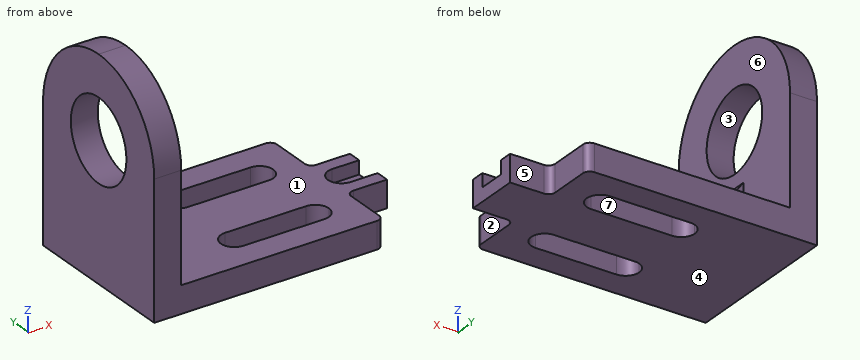
```python
from build123d import *

# Parameters (mm, degrees)
F1_DEPTH = 25.4
F2_DEPTH = 12.7
F3_R     = 38.1
F4_DEPTH = 25.4
F6_START = -63.5
F6_DEPTH = 25.4


with BuildPart() as f1:
    # F0 (on Top) → F1 (new body)
    with BuildSketch(Plane.XY):
        with BuildLine():
            Line((88.9, -38.1), (0, -38.1))
            Line((0, -38.1), (0, -114.3))
            Line((0, -114.3), (88.9, -114.3))
            ThreePointArc((88.9, -114.3), (92.6197438789, -105.3197438789), (101.6, -101.6))
            Line((101.6, -101.6), (177.8, -101.6))
            ThreePointArc((177.8, -101.6), (186.7802561211, -105.3197438789), (190.5, -114.3))
            Line((190.5, -114.3), (215.9, -114.3))
            Line((215.9, -114.3), (215.9, -107.95))
            ThreePointArc((215.9, -107.95), (217.7598719395, -103.4598719395), (222.25, -101.6))
            Line((222.25, -101.6), (254, -101.6))
            Line((254, -101.6), (254, -88.9))
            Line((254, -88.9), (228.6, -88.9))
            ThreePointArc((228.6, -88.9), (219.6197438789, -85.1802561211), (215.9, -76.2))
            ThreePointArc((215.9, -76.2), (219.6197438789, -67.2197438789), (228.6, -63.5))
            Line((228.6, -63.5), (254, -63.5))
            Line((254, -63.5), (254, -50.8))
            Line((254, -50.8), (222.25, -50.8))
            ThreePointArc((222.25, -50.8), (217.7598719395, -48.9401280605), (215.9, -44.45))
            Line((215.9, -44.45), (215.9, -38.1))
            Line((215.9, -38.1), (190.5, -38.1))
            ThreePointArc((190.5, -38.1), (186.7802561211, -47.0802561211), (177.8, -50.8))
            Line((177.8, -50.8), (101.6, -50.8))
            ThreePointArc((101.6, -50.8), (92.6197438789, -47.0802561211), (88.9, -38.1))
        make_face()
        with BuildLine():
            Line((209.55, 0), (0, 0))
            Line((0, 0), (0, -38.1))
            Line((0, -38.1), (88.9, -38.1))
            ThreePointArc((88.9, -38.1), (92.6197438789, -29.1197438789), (101.6, -25.4))
            Line((101.6, -25.4), (177.8, -25.4))
            ThreePointArc((177.8, -25.4), (186.7802561211, -29.1197438789), (190.5, -38.1))
            Line((190.5, -38.1), (215.9, -38.1))
            Line((215.9, -38.1), (215.9, -6.35))
            ThreePointArc((215.9, -6.35), (214.0401280605, -1.8598719395), (209.55, 0))
        make_face()
        with BuildLine():
            Line((88.9, -114.3), (0, -114.3))
            Line((0, -114.3), (0, -152.4))
            Line((0, -152.4), (209.55, -152.4))
            ThreePointArc((209.55, -152.4), (214.0401280605, -150.5401280605), (215.9, -146.05))
            Line((215.9, -146.05), (215.9, -114.3))
            Line((215.9, -114.3), (190.5, -114.3))
            ThreePointArc((190.5, -114.3), (186.7802561211, -123.2802561211), (177.8, -127))
            Line((177.8, -127), (101.6, -127))
            ThreePointArc((101.6, -127), (92.6197438789, -123.2802561211), (88.9, -114.3))
        make_face()
    extrude(amount=F1_DEPTH)

    # F0 (on Top) → F2 (join)
    with BuildSketch(Plane.XY):
        with BuildLine():
            Line((254, -88.9), (254, -63.5))
            Line((254, -63.5), (228.6, -63.5))
            ThreePointArc((228.6, -63.5), (219.6197438789, -67.2197438789), (215.9, -76.2))
            ThreePointArc((215.9, -76.2), (219.6197438789, -85.1802561211), (228.6, -88.9))
            Line((228.6, -88.9), (254, -88.9))
        make_face()
    extrude(amount=F2_DEPTH)

    # F3 (on face) → F4 (join)
    with BuildSketch(Plane(origin=(0, 0, 0), x_dir=(0, -1, 0), z_dir=(-1, 0, 0))):
        with BuildLine():
            Line((0, 127), (0, 25.4))
            Line((0, 25.4), (152.4, 25.4))
            Line((152.4, 25.4), (152.4, 127))
            ThreePointArc((152.4, 127), (130.0815367264, 180.8815367264), (76.2, 203.2))
            ThreePointArc((76.2, 203.2), (22.3184632736, 180.8815367264), (0, 127))
        make_face()
        with Locations((76.2, 127)):
            Circle(F3_R, mode=Mode.SUBTRACT)
    extrude(amount=-F4_DEPTH)

    # F5 (on face) → F6 (join)
    with BuildSketch(Plane.XZ.offset(152.4).offset(F6_START)):
        Polygon((25.4, 76.2), (25.4, 25.4), (63.5, 25.4), align=None)
    extrude(amount=-F6_DEPTH)


solid = f1.part
```
Can you work these out from the model? Positions are in its coordinate system, mm. Face numbers are marked on the shaded views. A direction names the side the tool comes from. Round coordinates to 2 decimals unless told otherwise and drop trailing zeros. Loops run counter-clockwise (first coordinate to the right, second up) from the corner with the lowest first, then second, coordinate; pieces in that order, holes last. Notation, with made-up numbers: M 42,47.5 L 49,47.5 A18 ccw 49,76.5 Z; hole C -32.75,42.25 d5. An arc over 180 degrees is marked long. Answer as a JSON object with one key per item and string values. Group by question number.
Q1. Will these pins go through, and if not, where does the flat tip stop? pin 1 (12.5 mm diameter, centred on y = -28.5, z = 9, fed in from +X); pin 2 (10 mm diameter, centred on x = 245, z = 18, fed in from +Y); pin 3 (20.5 mm diameter, centred on x = 246, z = 15, fed in from -Y).
Q2. Imagine slicing it at B-B, the plane z = 41. Please give me the cut outline in (x, y), then the cut area to 3 significant figures.
Q3. Imagine slicing it at D-D, the plane z = 117. Please give me the cut outline in (x, y), then the cut area to 3 significant figures.
Q4. We'd pull the mould along Z, two halves only. Please class the marked faces 1, 2, 3 and 4: +Z half, -Z half, draft (parallel to the pull), parting line (faces both ways), or undercut.
Q5. Please list where these lines run through material, in increasing order: L1, parallel to Z at x = 8, y = -76; L2, parallel to X at y = -118, z = 173.5; L3, parallel to Z at x = 223.5, y = -67.5.
Q6. Imagine slicing it at A-A, the plane z = 19. Please give me the cut outline in (x, y).
Q7. Imagine slicing it at C-C, the plane x = 187.5. Please give me the cut outline in (y, z).
Q8. On a 3-axis mill with a long thin cutter (end or side, diameter ignored), from which of +Z, -Z, +X, -X, +Y, -Y can I reach the whole of each face in a straight line? I mean the marked faces 5, 6 and 7. Say none if no direction works.
Findings:
{
 "1": {"pin 1": "stops at x = 215.9", "pin 2": "stops at y = -50.8", "pin 3": "stops at y = -101.6"},
 "2": {"outline": "M 0,-152.4 L 25.4,-152.4 L 25.4,-88.9 L 51.8,-88.9 L 51.8,-63.5 L 25.4,-63.5 L 25.4,0 L 0,0 Z", "area": "4,540 mm2"},
 "3": {"outline": "M 0,-152.4 L 25.4,-152.4 L 25.4,-112.96 L 0,-112.96 Z; M 0,-39.44 L 25.4,-39.44 L 25.4,0 L 0,0 Z", "area": "2,000 mm2"},
 "4": {"face 1": "+Z half", "face 2": "draft", "face 3": "undercut", "face 4": "-Z half"},
 "5": {"L1": "z = 0 to 88.9, 165.1 to 203.2", "L2": "x = 0 to 25.4", "L3": "z = 0 to 12.7"},
 "6": {"outline": "M 0,-152.4 L 209.55,-152.4 A6.35 ccw 215.9,-146.05 L 215.9,-107.95 A6.35 cw 222.25,-101.6 L 254,-101.6 L 254,-88.9 L 228.6,-88.9 A12.7 cw 228.6,-63.5 L 254,-63.5 L 254,-50.8 L 222.25,-50.8 A6.35 cw 215.9,-44.45 L 215.9,-6.35 A6.35 ccw 209.55,0 L 0,0 Z; hole M 101.6,-127 L 177.8,-127 A12.7 ccw 177.8,-101.6 L 101.6,-101.6 A12.7 ccw Z; hole M 101.6,-50.8 L 177.8,-50.8 A12.7 ccw 177.8,-25.4 L 101.6,-25.4 A12.7 ccw Z"},
 "7": {"outline": "M -152.4,0 L -122.5,0 L -122.5,25.4 L -152.4,25.4 Z; M -106.1,0 L -46.3,0 L -46.3,25.4 L -106.1,25.4 Z; M -29.9,0 L 0,0 L 0,25.4 L -29.9,25.4 Z"},
 "8": {"face 5": "+Z, -Z, +X, +Y", "face 6": "+Z, +X", "face 7": "+Z, -Z"}
}
